from build123d import *

# Parameters (mm, degrees)
EXTRUDE_1_DEPTH = 4
SKETCH_2_R      = 3.75
EXTRUDE_2_DEPTH = 2
SKETCH_3_R      = 2.25
EXTRUDE_3_DEPTH = 1.5
SKETCH_4_W      = 36
SKETCH_4_H      = 4.5
EXTRUDE_4_DEPTH = 0.2


with BuildPart() as part:
    # Эскиз1 → Бобышка-Вытянуть1 (new body)
    with BuildSketch(Plane.XY):
        with BuildLine():
            Line((11.456832295, 0), (6, 0))
            Line((6, 0), (6, -8))
            Line((6, -8), (11.456832295, -8))
            ThreePointArc((11.456832295, -8), (11.863587803, -6.01835518), (12, -3.999999921))
            ThreePointArc((12, -3.999999921), (11.863587792, -1.981644742), (11.456832295, 0))
        make_face()
        with BuildLine():
            Line((6, -8), (6, 0))
            Line((6, 0), (0.543167705, 0))
            ThreePointArc((0.543167705, 0), (0.136412203, -1.981644781), (0, -4))
            ThreePointArc((0, -4), (0.136412203, -6.018355219), (0.543167705, -8))
            Line((0.543167705, -8), (6, -8))
        make_face()
    extrude(amount=EXTRUDE_1_DEPTH)

    # Эскиз2 → Бобышка-Вытянуть2 (add)
    with BuildSketch(Plane.XY.offset(4)):
        with Locations((6, -4)):
            Circle(SKETCH_2_R)
    extrude(amount=EXTRUDE_2_DEPTH)

    # Эскиз3 → Бобышка-Вытянуть3 (add)
    with BuildSketch(Plane.XY.offset(6)):
        with Locations((6, -4)):
            Circle(SKETCH_3_R)
    extrude(amount=EXTRUDE_3_DEPTH)

    # Эскиз4 → Бобышка-Вытянуть4 (add)
    with BuildSketch(Plane(origin=(0, 0, 3), x_dir=(-1, 0, 0), z_dir=(0, 0, -1))):
        with Locations((-6, -4)):
            Rectangle(SKETCH_4_W, SKETCH_4_H)
    extrude(amount=EXTRUDE_4_DEPTH)


solid = part.part
Can you work these out from the model? Positions are in its coordinate system, mm. A direction names the side the tool comes from. Coordinates: 2 decimals unless noted, no trailing zeros. Order: outer loops, then holes, each group sorted by start corner. A loop starts at its lowest first (then second) coordinate and runs counter-clockwise, first axis right, second up. Notation, with made-up numbers: (49.5, 36.25) - (98.5, 36.25) arc R5 cw to (98.5, 41.25) - close; hole circle Ø1 at (55.5, 88.25). An arc over 180 degrees is marked (long way). Answer as a JSON object with one key per item and string values. Group by question number.
Q1. Imagine slicing it at C-C (y = -2.5). Please give me the cut outline in (x, z), and give its area (3 significant figures).
Q2. Imagine slicing it at B-B (z = 2.25). Please give me the cut outline in (x, y), and give its area (3 significant figures).
Q3. I need wall thicknesses on line 1 (X direction, y = -3.75, z = 2.5); line 2 (Z direction, x = 9, y = -2.25); line 3 (Z direction, x = 16, y = -5). Which ranges of each line are inside material? Lowest first, please. Write a range as from..to.
Q4. Imagine slicing it at D-D (z = 4.75). Please give me the cut outline in (x, y).
Q5. Imagine slicing it at A-A (x = 6). Please give me the cut outline in (y, z), and give its area (4 significant figures).
Q6. Will these pins go through, and if not, where does the flat tip stop? P1, Ø1.4, axis at x = -6, y = -4, coming from the +Z side; P2, Ø3, axis at x = 12.5, y = -7, coming from the +Z side; P3, Ø2, axis at x = -3, y = -1.5, coming from the -Z side.
Q7. On a 3-axis mill with a long thin cutter (end or side, diameter ignored), from which of +Z, -Z, +X, -X, +Y, -Y can I reach the whole of each face in a straight line? I mean faces 1 (the face through (6, -8, 2)), 2 (the face through (8, -6, 6)). Say none if no direction works.
Determined:
{
 "1": {"outline": "(-12, 2.8) - (0.08, 2.8) - (0.08, 0) - (11.92, 0) - (11.92, 2.8) - (24, 2.8) - (24, 3) - (11.92, 3) - (11.92, 4) - (9.44, 4) - (9.44, 6) - (7.68, 6) - (7.68, 7.5) - (4.32, 7.5) - (4.32, 6) - (2.56, 6) - (2.56, 4) - (0.08, 4) - (0.08, 3) - (-12, 3) - close", "area": "71.0 mm2"},
 "2": {"outline": "(0.54, -8) - (11.46, -8) arc R15 ccw to (11.46, 0) - (0.54, 0) arc R15 ccw to start", "area": "93.1 mm2"},
 "3": {"line 1": "x = 0..12", "line 2": "z = 0..6", "line 3": "z = 2.8..3"},
 "4": {"outline": "circle Ø7.5 at (6, -4)"},
 "5": {"outline": "(-8, 0) - (0, 0) - (0, 4) - (-0.25, 4) - (-0.25, 6) - (-1.75, 6) - (-1.75, 7.5) - (-6.25, 7.5) - (-6.25, 6) - (-7.75, 6) - (-7.75, 4) - (-8, 4) - close", "area": "53.75 mm2"},
 "6": {"P1": "stops at z = 3", "P2": "stops at z = 4", "P3": "stops at z = 2.8"},
 "7": {"face 1": "+Z, -Z, +X, -X, -Y", "face 2": "+Z"}
}
